Print and shaded views of the part. All mm, measured from the part's lowest x, y and z. A direction names the side the tool comes from. Coordinates: 2 decimals unless noted, no trailing zeros. Order: outer loops, then holes, each group sorted by start corner. A loop starts at its lowest first (then second) coordinate and runs counter-clockwise, first axis right, second up.
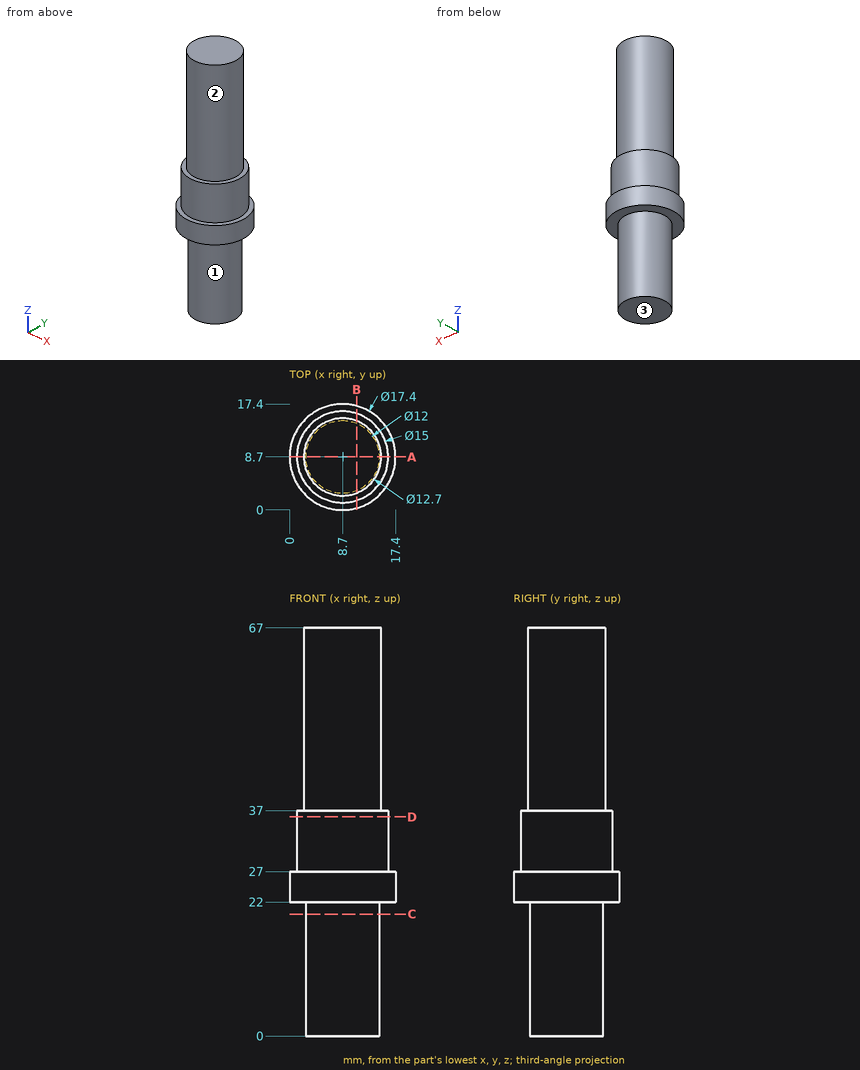
Q1. Which spindle directions (+Z, -Z, +X, -X, +Y, -Y) get a long thin tool onto all of the face, cutting with end or side? Do the marked faces 1, 2 and 3. Say none if no direction does.
Established:
face 1: -Z
face 2: +Z
face 3: -Z, +X, -X, +Y, -Y
Q2. Cut at C-C, the plane z = 20. List the corners of the cut face in (x, y).
Established:
outline: circle Ø12 at (8.7, 8.7)
Q3. Drop flat-ended pins along their axis: P1, Ø1, axis at y = 9.5, z = 31.5, coming from the -X side; P2, Ø1.5, axis at x = 3, z = 12.5, coming from the +Y side; P3, Ø3, axis at x = 6.5, z = 25, coming from the -Y side. Give the stop position or say it passes through.
Established:
P1: stops at x = 1.21
P2: stops at y = 12.09
P3: stops at y = 0.03
Q4. Cut at A-A, the plane y = 8.7. List the corners of the cut face in (x, z), plus the area to 3 significant figures.
Established:
outline: (0, 22) - (2.7, 22) - (2.7, 0) - (14.7, 0) - (14.7, 22) - (17.4, 22) - (17.4, 27) - (16.2, 27) - (16.2, 37) - (15.05, 37) - (15.05, 67) - (2.35, 67) - (2.35, 37) - (1.2, 37) - (1.2, 27) - (0, 27) - close
area: 882 mm2
Q5. Probe line 1 (Z direction, x = 10.5, y = 1); line 2 (Y direction, x = 9, z = 19.5); line 3 (Z direction, x = 14.75, y = 8.5). List the from-to ranges inside material, lowest first.
Established:
line 1: z = 22 to 27
line 2: y = 2.71 to 14.69
line 3: z = 22 to 67
Q6. Cut at D-D, the plane z = 36. List the corners of the cut face in (x, y), plus the area to 3 significant figures.
Established:
outline: circle Ø15 at (8.7, 8.7)
area: 177 mm2
Q7. Cut at B-B, the plane x = 11. List the corners of the cut face in (y, z).
Established:
outline: (0.31, 22) - (3.16, 22) - (3.16, 0) - (14.24, 0) - (14.24, 22) - (17.09, 22) - (17.09, 27) - (15.84, 27) - (15.84, 37) - (14.62, 37) - (14.62, 67) - (2.78, 67) - (2.78, 37) - (1.56, 37) - (1.56, 27) - (0.31, 27) - close
